Model file for the job. Use its own axes, mm. A direction names the side the tool comes from. Round coordinates to 2 decimals unless told otherwise and drop trailing zeros. Write each loop counter-clockwise with the first axis right and the second up, starting at its lowest first coordinate (ties: lowest second). Pieces come first, ordered by that corner, then holes. Notation, with made-up numbers: (68, 59.25) - (113, 59.25) arc R30 ccw to (113, 87.25) - close; hole circle Ø11 at (27.5, 72). An arc over 180 degrees is marked (long way). Answer as a JSON object with one key per item and string values. Group by question number.
from build123d import *

# Parameters (mm, degrees)
BOSS_EXTRUDE1_DEPTH = 4
BOSS_EXTRUDE1_DRAFT = 1
SHELL1_T            = -0.5
SKETCH2_R           = 2
BOSS_EXTRUDE2_DEPTH = 5.5
BOSS_EXTRUDE2_TAPER = 1.5
RIB1_START          = -0.25
RIB1_DEPTH          = 0.5
CIRPATTERN1_COUNT   = 4


# Read off the part's stored shape, not the designer's step: Rib1
with BuildPart() as part:
    # Sketch1 → Boss-Extrude1 (with draft: the straight prism first)
    with BuildSketch(Plane(origin=(0, 0, 0), x_dir=(1, 0, 0), z_dir=(0, 1, 0))):
        with BuildLine():
            Line((-7.5, -6.375), (7.5, -6.375))
            ThreePointArc((7.5, -6.375), (8.207106781, -6.082106781), (8.5, -5.375))
            Line((8.5, -5.375), (8.5, 5.375))
            ThreePointArc((8.5, 5.375), (8.207106781, 6.082106781), (7.5, 6.375))
            Line((7.5, 6.375), (-7.5, 6.375))
            ThreePointArc((-7.5, 6.375), (-8.207106781, 6.082106781), (-8.5, 5.375))
            Line((-8.5, 5.375), (-8.5, -5.375))
            ThreePointArc((-8.5, -5.375), (-8.207106781, -6.082106781), (-7.5, -6.375))
        make_face()
    extrude(amount=-BOSS_EXTRUDE1_DEPTH)
    # Boss-Extrude1: the draft: its side faces are tilted about the plane it starts from
    boss_extrude1_sides = [part.faces().sort_by_distance(p)[0] for p in [
        (0, -2, 6.375),
        (8.207106781, -2, 6.082106781),
        (8.5, -2, 0),
        (8.207106781, -2, -6.082106781),
        (0, -2, -6.375),
        (-8.207106781, -2, -6.082106781),
        (-8.5, -2, 0),
        (-8.207106781, -2, 6.082106781),
    ]]
    draft(boss_extrude1_sides, Plane(origin=(0, 0, 0), x_dir=(1, 0, 0), z_dir=(0, 1, 0)), BOSS_EXTRUDE1_DRAFT)

    # Shell1
    shell1_openings = [part.faces().sort_by_distance(p)[0] for p in [
        (0, -4, 0),
    ]]
    offset(amount=SHELL1_T, openings=shell1_openings, kind=Kind.INTERSECTION)

    # Sketch2 → Boss-Extrude2 (add)
    with BuildSketch(Plane.XZ.offset(0.5)):
        Circle(SKETCH2_R)
    extrude(amount=BOSS_EXTRUDE2_DEPTH, taper=BOSS_EXTRUDE2_TAPER)

    # Rib1 outline → Rib1 (add)
    with BuildSketch(Plane.XY.offset(RIB1_START)):
        Polygon((-2.396376072, -4.46378352), (-1, -4.46378352), (-1, 0), (-2.893975097, 0), (-2.838237736, -0.5), align=None)
    rib1 = extrude(amount=RIB1_DEPTH)

    # CirPattern1: Rib1 ×4 about axis
    cirpattern1_axis = Axis((0, 0, 0), (0, 1, 0))
    for i in range(1, CIRPATTERN1_COUNT):
        add(rib1.rotate(cirpattern1_axis, i * 360 / CIRPATTERN1_COUNT))


solid = part.part
(1) Drill centre lines: line 1 (X direction, y = -1, z = -0.75); line 2 (X direction, y = -3.5, z = -1.5); line 3 (Z direction, x = 5.25, y = -3.75). Where is each one in solid material? Low to high. Write a range as from..to.
(2) Slice it at C-C (z = 3.5). Write the cut outline in (x, y).
(3) Pull direction Z, two halves, no side cores. Call faces 1 (the conical face through (8.24, -1.97, -6.1)), 2 (the flat face through (2.3, -2.5, -0.25)), 3 (the conical face through (1.78, -3.29, -0.74)), 4 (the conical face through (-8.24, -1.97, 6.1)): pulls with the +Z half, pulls with the -Z half, needs draft (parallel to the pull), parting line crosses it, or undercut.
(4) Slice it at A-A (y = -1). Count the separate pieces of the cut face and the enclosed holes in it, then the cut area to 3 significant figures.
(5) Slice it at B-B (x = 6.5). Write the cut outline in (y, z) (3 decimals), then the cut area to 3 significant figures.
(6) 3-axis set-ups, long thin cutter, end or side, ignore diameter. For faces 5 (the conical face through (-8.223, -1.972, -6.114)), 6 (the flat face through (2.3, -2.5, 0.25)), 7 (the flat face through (0, 0, 0)): which of +Z, -Z, +X, -X, +Y, -Y reach the whole face in a straight line?
(7) Flat gauge pins, fed straight in: pin 1 (0.5 mm diameter, centred on y = -2, z = 2.5, fed in from +X); pin 2 (0.5 mm diameter, centred on x = -2.5, y = -2, fed in from -Z); pin 3 (1.5 mm diameter, centred on x = 1.5, z = 4.5, fed in from -Y); pin 4 (1 mm diameter, centred on x = 6.5, y = -5, fed in from -Z). Where does each tip first touch, or does it go through?
Answer:
{
 "1": {"line 1": "-8.52..-8.02, -1.84..1.84, 8.02..8.52", "line 2": "-8.56..-8.06, -1.2..1.2, 8.06..8.56", "line 3": "-6.44..-5.94, 5.94..6.44"},
 "2": {"outline": "(-8.57, -4) - (-8.07, -4) - (-8.01, -0.5) - (8.01, -0.5) - (8.07, -4) - (8.57, -4) - (8.5, 0) - (-8.5, 0) - close"},
 "3": {"face 1": "pulls with the -Z half", "face 2": "undercut", "face 3": "undercut", "face 4": "pulls with the +Z half"},
 "4": {"separate pieces": "2", "enclosed holes": "1", "area": "42.2 mm²"},
 "5": {"outline": "(-4, -6.445) - (0, -6.375) - (0, 6.375) - (-4, 6.445) - (-4, 5.945) - (-0.5, 5.884) - (-0.5, -5.884) - (-4, -5.945) - close", "area": "9.88 mm²"},
 "6": {"face 5": "-Z, -X, +Y", "face 6": "-Y", "face 7": "+Z, -Z, +X, -X, +Y"},
 "7": {"pin 1": "x = 8.54", "pin 2": "z = -6.41", "pin 3": "y = -0.5", "pin 4": "through"}
}
